The model under review builds one solid part; all positions refer to its coordinate system, in mm. Coordinates: 2 decimals unless noted, no trailing zeros. Loops run counter-clockwise (first coordinate to the right, second up) from the corner with the lowest first, then second, coordinate; pieces in that order, holes last. Notation, with made-up numbers: (-0.5, -27) - (13.5, -27) arc R9 ccw to (13.5, -10) - close; hole circle Ø2 at (-4.75, -15.75). An arc over 180 degrees is marked (long way). One line per item, written item: value. Start each with the question number.
1. We need section A-A, the plane y = -21. Give the boundary of the cut face in (x, z) (3 decimals).
2. We need section B-B, the plane y = 8. Count the separate pieces of the cut face and the enclosed holes in it, then the cut area to 3 significant figures.
3. Insertion check: P1, Ø5, axis at x = -14, y = 5.5, coming from the -Z side; P2, Ø12, axis at y = 14.5, z = -24.5, coming from the +X side. Each pin has a flat end and moves straight along its axis. Give the tip position at first contact, or say it passes through.
4. To check wall thickness, follow line 1 (Z direction, x = 32.5, y = -8) (3 decimals); line 2 (X direction, y = 5, z = -6.5); line 3 (X direction, y = 35.5, z = -106). State the ranges of each line that lie inside material, in increasing order.
5. We need section C-C, the plane y = 66. Give the boundary of the cut face in (x, z) (3 decimals).
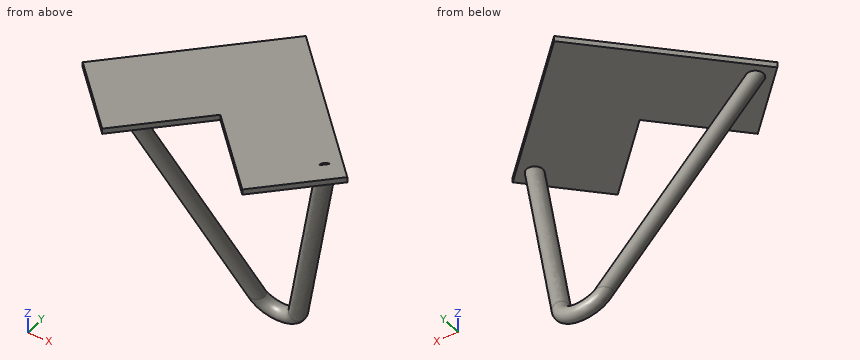
from build123d import *

# Parameters (mm, degrees)
F1_DEPTH = 3.175
F6_R     = 4.7625


with BuildPart() as f1:
    # F0 (on Top) → F1 (new body)
    with BuildSketch(Plane.XY):
        Polygon((76.332177, 0), (0, 76.332177), (-76.332177, 0), (-40.411153, -35.921024), (0, 4.490128), (40.411153, -35.921024), align=None)
    extrude(amount=F1_DEPTH)

    # F7: sweep along a path in F5
    with BuildLine(Plane(origin=(0, 0, 0), x_dir=(1, 0, 0), z_dir=(0, -0.939693, -0.34202))) as f7_path:
        Line((-63.632177, 0), (-12.038401, -153.526296))
        ThreePointArc((-12.038401, -153.526296), (0, -162.180693), (12.038401, -153.526296))
        Line((12.038401, -153.526296), (63.632177, 0))
    # F6 (on face) → F7 (sweep)
    with BuildSketch(Plane(origin=(0, 0, 0), x_dir=(1, 0, 0), z_dir=(0, 0, -1))):
        with Locations((-63.632177, 0)):
            Circle(F6_R)
    sweep(path=f7_path.line)


solid = f1.part
Findings below:
1. outline: (-55.332, 0) - (-25.49, 0) - (-25.49, 3.175) - (-55.332, 3.175) - close; (25.49, 0) - (55.332, 0) - (55.332, 3.175) - (25.49, 3.175) - close
2. separate pieces: 3
2. enclosed holes: 0
2. area: 825 mm2
3. P1: z = 0
3. P2: x = 60.47
4. line 1: 0 to 3.175
4. line 2: -65.28 to -57.34, 57.34 to 65.28
4. line 3: -29.36 to -22.09, 22.09 to 29.36
5. outline: (-10.332, 0) - (10.332, 0) - (10.332, 3.175) - (-10.332, 3.175) - close
